Source: CAD feature listing. Evaluate the final solid. Frame: model axes, mm. Face numbers are marked on the shaded views. A direction names the side the tool comes from. Round coordinates to 2 decimals unless told otherwise and drop trailing zeros. Order: outer loops, then holes, each group sorted by start corner. A loop starts at its lowest first (then second) coordinate and runs counter-clockwise, first axis right, second up. Notation, with made-up numbers: (75.25, 72) - (79.25, 72) arc R17 ccw to (79.25, 101) - close; hole circle Ø9 at (43, -39.5). An arc over 180 degrees is marked (long way). Return JSON: item names as keys, results as strings. Group by question number.
1) Access query for the marked faces 4, 5 and 6. Directions: +Z, -Z, +X, -X, +Y, -Y. A direction counts if a zero-diameter tool reaches every point of the face in a straight line with its end or side. Return the directions, or none.
2) Section D-D, the plane x = 258.5. Return loops of the section in (y, z).
3) Section A-A, the plane x = 169.5. Return loops of the section in (y, z), plus the area to 3 significant figures.
4) Ray query, line 1 (Z direction, x = 135, y = -10.5); line 2 (X direction, y = -13, z = 30.5); line 3 (Z direction, x = 170.5, y = -15.5). Return the intervals inside material, ascending. Write a range as from..to.
5) Contact query for flat-ended pins moving along their axis: P1, Ø1, axis at x = 38.5, y = -17, coming from the +Z side; P2, Ø12, axis at x = 127.5, z = 123, coming from the -Y side; P3, Ø1.5, axis at x = 11.5, y = -13.5, coming from the +Z side; P4, Ø2, axis at x = 207, z = 69.5, coming from the +Y side. Output: stop coordinate, or through.
6) Section B-B, the plane z = 15. Return loops of the section in (x, y).
7) Mould query, pull axis Z, two halves, no side actions, for the marked faces 1, 2 and 3. Classes: pulls with the +Z half, pulls with the -Z half, needs draft (parallel to the pull), parting line crosses it, or undercut.
8) Section C-C, the plane x = 58. Return loops of the section in (y, z).
```python
from build123d import *

# Parameters (mm, degrees)
PAD_DEPTH    = 20
SKETCH001_R  = 2.15
POCKET_DEPTH = 47
CHAMFER_SIZE = 1.5
PAD001_DEPTH = 4


with BuildPart() as part:
    # Sketch → Pad (new body)
    with BuildSketch(Plane.XZ):
        with BuildLine():
            Line((4.0390093024, 42.5746936035), (2.6558476721, 42.7938363759))
            ThreePointArc((2.9062224976, 44.3741250985), (1.9908907236, 43.70916815), (2.6558476721, 42.7938363759))
            Line((2.9062224976, 44.3741250985), (5.030422984, 44.0375749994))
            Line((5.030422984, 44.0375749994), (5.030422984, 45.679507745))
            ThreePointArc((6.630422984, 45.679507745), (5.830422984, 46.479507745), (5.030422984, 45.679507745))
            Line((6.630422984, 45.679507745), (6.630422984, 44.1665554588))
            Line((6.630422984, 44.1665554588), (8.4415504736, 45.4111549307))
            Line((8.4415504736, 45.4111549307), (9.4473057083, 46.1365999544))
            ThreePointArc((10.36219, 44.864349), (10.5417900599, 45.9585758488), (9.4473057083, 46.1365999544))
            Line((10.36219, 44.864349), (7.8490460164, 43.0626150502))
            Line((7.8490460164, 43.0626150502), (5.6390093024, 41.5438867756))
            Line((5.6390093024, 41.5438867756), (7.0549059293, 39.4834895465))
            Line((7.0549059293, 39.4834895465), (12.3295228359, 43.1081849113))
            Line((12.3295228359, 43.1081849113), (38.9483794216, 4.3727170031))
            Line((134.8804744114, 70.2968639515), (38.9483794216, 4.3727170031))
            Line((119.3056115155, 92.9612334723), (134.8804744114, 70.2968639515))
            Line((134.9646304571, 103.7220478367), (119.3056115155, 92.9612334723))
            Line((142.0441135916, 93.4200616909), (134.9646304571, 103.7220478367))
            Line((237.9762085814, 159.3442086393), (142.0441135916, 93.4200616909))
            Line((219.8527317571, 185.7172931726), (237.9762085814, 159.3442086393))
            Line((225.1273486637, 189.3419885375), (219.8527317571, 185.7172931726))
            Line((223.7114520368, 191.4023857666), (225.1273486637, 189.3419885375))
            Line((218.4368351302, 187.7776904018), (223.7114520368, 191.4023857666))
            Line((218.4368351302, 187.7776904018), (217.5306612889, 189.0963446284))
            Line((217.5306612889, 189.0963446284), (221.3848485497, 191.7449264963))
            Line((221.3848485497, 191.7449264963), (219.3793189808, 192.1708640962))
            ThreePointArc((219.6286165225, 193.3446829646), (218.9170583175, 192.8824223013), (219.3793189808, 192.1708640962))
            Line((219.6286165225, 193.3446829646), (221.2482697259, 193.0006984087))
            Line((221.2482697259, 193.0006984087), (222.3395205202, 195.3340273515))
            ThreePointArc((223.4265178948, 194.8256606455), (223.1372025604, 195.6233426858), (222.3395205202, 195.3340273515))
            Line((223.4265178948, 194.8256606455), (222.4583086449, 192.755420993))
            Line((222.4583086449, 192.755420993), (225.3597698201, 192.5351030681))
            Line((225.3597698201, 192.5351030681), (227.2058553447, 189.8486996773))
            Line((227.2058553447, 189.8486996773), (225.1628423907, 186.850988034))
            Line((225.1628423907, 186.850988034), (229.8793547275, 185.6901341722))
            ThreePointArc((229.5925630359, 184.5249086465), (230.3185716445, 184.9641255636), (229.8793547275, 185.6901341722))
            Line((229.5925630359, 184.5249086465), (227.4493724265, 185.0524024636))
            Line((227.4493724265, 185.0524024636), (226.9439351411, 182.6613604036))
            ThreePointArc((225.7710395828, 182.6559948849), (226.3596521523, 182.1854572192), (226.9439351411, 182.6613604036))
            Line((225.7710395828, 182.6559948849), (226.2736384812, 185.0336095568))
            Line((226.2736384812, 185.0336095568), (223.7973399844, 183.331907264))
            Line((223.7973399844, 183.331907264), (226.0061387224, 180.1176875865))
            Line((226.0061387224, 180.1176875865), (232.1873304099, 184.3653774672))
            Line((232.1873304099, 184.3653774672), (247.1063382508, 153.1208066582))
            Line((247.1063382508, 153.1208066582), (245.3756045783, 151.9314534916))
            Line((226.9968612942, 139.3016555797), (245.3756045783, 151.9314534916))
            Line((222.4093562231, 145.9773426022), (226.9968612942, 139.3016555797))
            Line((225.5411600114, 148.1295054751), (222.4093562231, 145.9773426022))
            Line((229.2224912413, 142.7724726792), (225.5411600114, 148.1295054751))
            Line((232.2718791405, 144.867999687), (229.2224912413, 142.7724726792))
            Line((227.9109175296, 151.2140231529), (232.2718791405, 144.867999687))
            Line((214.9716229305, 142.3221923359), (227.9109175296, 151.2140231529))
            Line((219.3325845414, 135.9761688701), (214.9716229305, 142.3221923359))
            Line((222.3819724405, 138.0716958779), (219.3325845414, 135.9761688701))
            Line((218.7006412106, 143.4287286737), (222.3819724405, 138.0716958779))
            Line((220.3489589939, 144.5614459753), (218.7006412106, 143.4287286737))
            Line((224.9364640651, 137.8857589528), (220.3489589939, 144.5614459753))
            Line((216.5602719319, 132.1296736602), (224.9364640651, 137.8857589528))
            Line((214.1249297336, 135.6735568944), (216.5602719319, 132.1296736602))
            Line((214.1249297336, 135.6735568944), (161.5133638836, 99.5191020307))
            Line((161.5133638836, 99.5191020307), (229.6352159636, 0.3889306577))
            Line((290.6229739468, 42.2994708139), (229.6352159636, 0.3889306577))
            Line((294.258762918, 37.008710613), (290.6229739468, 42.2994708139))
            Line((296.3191601472, 38.4246072399), (294.258762918, 37.008710613))
            Line((292.4603634449, 44.0398858431), (296.3191601472, 38.4246072399))
            Line((292.4603634449, 44.0398858431), (293.7790176715, 44.9460596843))
            Line((293.7790176715, 44.9460596843), (296.6113530901, 40.8244762739))
            Line((296.6113530901, 40.8244762739), (297.055734393, 42.735476101))
            ThreePointArc((298.2789600102, 42.4510288783), (297.809570813, 43.2048652982), (297.055734393, 42.735476101))
            Line((298.2789600102, 42.4510288783), (297.7984698218, 40.3847478241))
            Line((297.7984698218, 40.3847478241), (300.0943558548, 39.8731393346))
            ThreePointArc((299.8212028325, 38.6473422227), (300.5706778996, 39.1236642674), (300.0943558548, 39.8731393346))
            Line((299.8212028325, 38.6473422227), (297.7654069564, 39.105449728))
            Line((297.7654069564, 39.105449728), (296.952983487, 36.4334515477))
            Line((296.952983487, 36.4334515477), (295.3914802195, 35.3603928297))
            Line((295.3914802195, 35.3603928297), (291.8734315191, 36.0212597001))
            Line((291.8734315191, 36.0212597001), (290.6278670782, 32.2423690465))
            ThreePointArc((289.4121870072, 32.3352401719), (289.9836654433, 31.8128324322), (290.6278670782, 32.2423690465))
            Line((289.4121870072, 32.3352401719), (290.1017184324, 34.427194448))
            Line((290.1017184324, 34.427194448), (287.5647756287, 35.1692737258))
            ThreePointArc((287.653171066, 36.3937007315), (287.1147629857, 35.8171659101), (287.5647756287, 35.1692737258))
            Line((287.653171066, 36.3937007315), (290.0713769403, 35.6863531059))
            Line((290.0713769403, 35.6863531059), (288.2375880383, 38.3548625865))
            Line((288.2375880383, 38.3548625865), (285.0350616215, 36.1290479439))
            Line((285.0350616215, 36.1290479439), (289.2827515022, 29.9478562564))
            Line((289.2827515022, 29.9478562564), (228.604015, -5.173139512))
            Line((37.917178458, -1.1893531666), (228.604015, -5.173139512))
            Line((9.1699343254, 31.1087265717), (37.917178458, -1.1893531666))
            Line((15.3511260129, 35.3564164524), (9.1699343254, 31.1087265717))
            Line((13.1423272749, 38.5706361299), (15.3511260129, 35.3564164524))
            Line((10.619338857, 36.8368487126), (13.1423272749, 38.5706361299))
            Line((12.4568191979, 36.8368487126), (10.619338857, 36.8368487126))
            ThreePointArc((12.4568191979, 35.2368487126), (13.2568191979, 36.0368487126), (12.4568191979, 36.8368487126))
            Line((10.2074312987, 35.2368487126), (12.4568191979, 35.2368487126))
            Line((10.2074312987, 33.9413217047), (10.2074312987, 35.2368487126))
            ThreePointArc((8.6074312987, 33.9413217047), (9.4074312987, 33.1413217047), (10.2074312987, 33.9413217047))
            Line((8.6074312987, 37.2714912173), (8.6074312987, 33.9413217047))
            Line((5.4065881459, 38.350772245), (8.6074312987, 37.2714912173))
            Line((4.0390093024, 40.3408579662), (5.4065881459, 38.350772245))
            Line((4.0390093024, 40.3408579662), (4.0390093024, 42.5746936035))
        make_face()
        Polygon((43.5674287195, 2.6934759176), (225.8145842591, -1.1139905174), (165.5793907768, 86.5396018361), align=None, mode=Mode.SUBTRACT)
    extrude(amount=PAD_DEPTH)

    # Sketch001 (on DatumPlane) → Pocket (cut)
    with BuildSketch(Plane(origin=(-5.1227490992, 0, 7.4545682568), x_dir=(-0.8241588917, 0, -0.5663586508), z_dir=(-0.5663586508, 0, 0.8241588917))):
        with Locations((-160.5, 9.9890381016)):
            Circle(SKETCH001_R)
    extrude(amount=-POCKET_DEPTH, mode=Mode.SUBTRACT)

    # Chamfer
    chamfer_edges = [part.edges().sort_by_distance(p)[0] for p in [
        (128.926695, -9.989038, 99.572803),
    ]]
    chamfer(chamfer_edges, length=CHAMFER_SIZE)

    # Sketch002 → Pad001 (join)
    with BuildSketch(Plane.XZ):
        Polygon((8.4415504736, 45.4111549307), (4.918851, 41.369339), (7.155737, 38.386826), (12.779469, 40.715076), (40.176517, 0.3632551244), (228.996323, 0.3632551244), (288.524261, 39.629669), (294.24765, 36.288891), (297.030212, 38.458557), (293.7790176715, 44.9460596843), (228.564316, 141.632828), (244.029541, 152.010803), (221.678513, 185.245819), (225.870392, 189.519104), (223.916901, 191.960983), (217.5306612889, 189.0963446284), (114.5322283976, 118.8000303552), (124.8392314819, 103.8013926071), (122.8612501419, 102.4421318452), (112.5542362208, 117.4407853631), align=None)
        Polygon((107.6796307846, 108.9964002019), (118.8935320696, 92.6780541469), (135.3767099029, 104.0052271621), (124.1628086179, 120.3235732171), (122.0199954996, 118.8510407251), (131.8746360228, 104.5106760101), (119.6770844261, 96.1285679789), (109.8224439029, 110.4689326938), align=None, mode=Mode.SUBTRACT)
    extrude(amount=PAD001_DEPTH)


solid = part.part
```
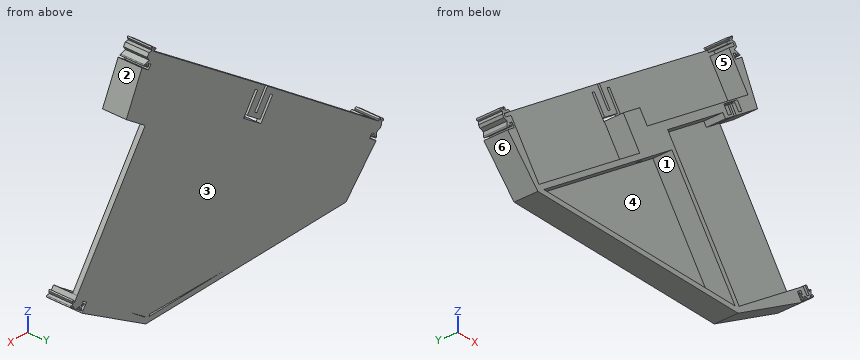
Geometry check:
{
 "1": {"face 4": "-Y", "face 5": "-X, -Y", "face 6": "-Z, -X, +Y, -Y"},
 "2": {"outline": "(-20, 12.13) - (0, 12.13) - (0, 97.25) - (-4, 97.25) - (-4, 20.22) - (-20, 20.22) - close"},
 "3": {"outline": "(-20, -3.94) - (0, -3.94) - (0, 0.06) - (-20, 0.06) - close; (-20, 80.83) - (-4, 80.83) - (-4, 0.36) - (0, 0.36) - (0, 156.32) - (-4, 156.32) - (-4, 112.29) - (-20, 112.29) - (-20, 105.01) - (-4, 105.01) - (-4, 87.9) - (-20, 87.9) - close", "area": "933 mm2"},
 "4": {"line 1": "-3.22..0.78, 65.53..83.25, 90.63..103.67", "line 2": "9.71..20.99, 76.97..84.03, 204.09..208.94, 273.45..288.9", "line 3": "-3.96..0.04, 79.38..86.44, 105.69..112.97"},
 "5": {"P1": "z = 5.75", "P2": "y = -4", "P3": "z = 43.05", "P4": "y = 0"},
 "6": {"outline": "(23.51, -20) - (31.65, -20) - (31.65, -4) - (54.41, -4) - (54.41, -20) - (61.48, -20) - (61.48, -4) - (214.74, -4) - (214.74, -20) - (219.59, -20) - (219.59, -4) - (250.9, -4) - (250.9, -20) - (263.46, -20) - (263.46, 0) - (23.51, 0) - close"},
 "7": {"face 1": "undercut", "face 2": "pulls with the +Z half", "face 3": "needs draft"},
 "8": {"outline": "(-20, -1.61) - (0, -1.61) - (0, 79.7) - (-4, 79.7) - (-4, 17.46) - (-20, 17.46) - (-20, 12.61) - (-4, 12.61) - (-4, 2.39) - (-20, 2.39) - close"}
}
